```python
from build123d import *

# Parameters (mm, degrees)
SKETCH1_R           = 9
SKETCH1_R_2         = 7
BOSS_EXTRUDE1_DEPTH = 20
BOSS_EXTRUDE2_DEPTH = 9
SKETCH3_R           = 9
SKETCH3_R_2         = 7
BOSS_EXTRUDE4_DEPTH = 20
SKETCH6_R           = 5
BOSS_EXTRUDE7_DEPTH = 10
BOSS_EXTRUDE8_START = 25
SKETCH6_3_R         = 5
BOSS_EXTRUDE8_DEPTH = 10


with BuildPart() as part:
    # Sketch1 → Boss-Extrude1 (new body)
    # profile 1 of 3: a face of its own
    with BuildSketch(Plane(origin=(0, 0, 0), x_dir=(0, 0, -1), z_dir=(1, 0, 0))):
        with BuildLine():
            Line((90, 9), (0, 9))
            ThreePointArc((0, 9), (6.363961031, 6.363961031), (9, 0))
            Line((9, 0), (81, 0))
            ThreePointArc((81, 0), (83.636038969, 6.363961031), (90, 9))
        make_face()
    # profile 2 of 3: a face of its own
    with BuildSketch(Plane(origin=(0, 0, 0), x_dir=(0, 0, -1), z_dir=(1, 0, 0))):
        Circle(SKETCH1_R)
        Circle(SKETCH1_R_2, mode=Mode.SUBTRACT)
    # profile 3 of 3: a face of its own
    with BuildSketch(Plane(origin=(0, 0, 0), x_dir=(0, 0, -1), z_dir=(1, 0, 0))):
        with Locations((90, 0)):
            Circle(SKETCH1_R)
        with Locations((90, 0)):
            Circle(SKETCH1_R_2, mode=Mode.SUBTRACT)
    extrude(amount=-BOSS_EXTRUDE1_DEPTH)

    # Sketch2 → Boss-Extrude2 (add)
    with BuildSketch(Plane(origin=(0, 9, 0), x_dir=(1, 0, 0), z_dir=(0, 1, 0))):
        Polygon((0, 62.5), (50, 62.5), (50, 52.5), (10, 52.5), (10, 37.5), (50, 37.5), (50, 27.5), (0, 27.5), align=None)
    extrude(amount=-BOSS_EXTRUDE2_DEPTH)

    # Sketch3 → Boss-Extrude4 (add)
    # profile 1 of 4: a face of its own
    with BuildSketch(Plane(origin=(50, 0, 0), x_dir=(0, 0, -1), z_dir=(1, 0, 0))):
        Circle(SKETCH3_R)
        Circle(SKETCH3_R_2, mode=Mode.SUBTRACT)
    # profile 2 of 4: a face of its own
    with BuildSketch(Plane(origin=(50, 0, 0), x_dir=(0, 0, -1), z_dir=(1, 0, 0))):
        with BuildLine():
            Line((27.5, 9), (0, 9))
            ThreePointArc((0, 9), (6.363961031, 6.363961031), (9, 0))
            Line((9, 0), (27.5, 0))
            Line((27.5, 0), (27.5, 9))
        make_face()
    # profile 3 of 4: a face of its own
    with BuildSketch(Plane(origin=(50, 0, 0), x_dir=(0, 0, -1), z_dir=(1, 0, 0))):
        with BuildLine():
            Line((90, 9), (52.5, 9))
            Line((52.5, 9), (52.5, 0))
            Line((52.5, 0), (81, 0))
            ThreePointArc((81, 0), (83.636038969, 6.363961031), (90, 9))
        make_face()
    # profile 4 of 4: a face of its own
    with BuildSketch(Plane(origin=(50, 0, 0), x_dir=(0, 0, -1), z_dir=(1, 0, 0))):
        with Locations((90, 0)):
            Circle(SKETCH3_R)
        with Locations((90, 0)):
            Circle(SKETCH3_R_2, mode=Mode.SUBTRACT)
    extrude(amount=-BOSS_EXTRUDE4_DEPTH)

    # Sketch6 → Boss-Extrude7 (add)
    with BuildSketch(Plane.XY.offset(-52.5)):
        with BuildLine():
            Line((10, 0), (24.4, -19.2))
            ThreePointArc((24.4, -19.2), (30, -22), (35.6, -19.2))
            Line((35.6, -19.2), (50, 0))
            Line((50, 0), (10, 0))
        make_face()
        with Locations((30, -15)):
            Circle(SKETCH6_R, mode=Mode.SUBTRACT)
    extrude(amount=-BOSS_EXTRUDE7_DEPTH)

    # Sketch6<3> → Boss-Extrude8 (add)
    with BuildSketch(Plane.XY.offset(-52.5).offset(BOSS_EXTRUDE8_START)):
        with BuildLine():
            Line((10, 0), (24.4, -19.2))
            ThreePointArc((24.4, -19.2), (30, -22), (35.6, -19.2))
            Line((35.6, -19.2), (50, 0))
            Line((50, 0), (10, 0))
        make_face()
        with Locations((30, -15)):
            Circle(SKETCH6_3_R, mode=Mode.SUBTRACT)
    extrude(amount=-BOSS_EXTRUDE8_DEPTH)


solid = part.part
```
Source: CAD feature listing. Evaluate the final solid. Frame: model axes, mm. A direction names the side the tool comes from. Give positions to 0.01 mm unless a question says otherwise; leave off trailing zeros. Loops run counter-clockwise (first coordinate to the right, second up) from the corner with the lowest first, then second, coordinate; pieces in that order, holes last. Notation, with made-up numbers: (-25, 49) -> (34, 49) arc R19 cw to (34, 65) -> close; hole circle Ø11 at (0.5, 36). An arc over 180 degrees is marked (long way). Put each result on its own line as item: value. Start each with the question number.
1) Cut plane B-B (z = -69). Return loops of the section in (x, y), then the cut area to 3 significant figures.
2) Contact query for flat-ended pins moving along their axis: P1, Ø9.5, axis at x = 34.5, y = -11.5, coming from the -Z side; P2, Ø14.5, axis at y = -1.5, z = -3, coming from the +X side; P3, Ø1.5, axis at x = 28, y = -6.5, coming from the +Z side; P4, Ø20.5, axis at x = 37, z = -74, coming from the -Y side. Output: stop coordinate, or through.
3) Reachability of faces 5 (the face through (0, 2, -9)), 6 (the face through (-8, 0, -44)), 7 (the face through (0, 2, -76)) from +Z, -Z, +X, -X, +Y, -Y: full face, straight path, thin tool, end or side. Return the list, or none.
4) Cut plane C-C (x = -2). Return loops of the section in (y, z).
5) Cut plane D-D (x = 23). Return loops of the section in (y, z), then the cut area to 3 significant figures.
6) Material intervals for probe 1 along X at (y, z) = (-7, -3); probe 2 along Y at (x, z) = (-14, -90); probe 3 along Z at (x, y) = (10.5, 4.5), sorted ascending.
7) Draft query along X for faces 1 (the face through (50, 4, -14)), 2 (the face through (25, -3, -62.5)), 3 (the face through (40, 0, -72)), 4 (the face through (17.099, -9.466, -57.43)). Return one class per face: released by +X, released by -X, zero draft, split by the parting line, or undercut.
8) Cut plane A-A (y = -18). Return loops of the section in (x, z), then the cut area to 3 significant figures.
Results are:
1. outline: (-20, 0) -> (0, 0) -> (0, 9) -> (-20, 9) -> close; (30, 0) -> (50, 0) -> (50, 9) -> (30, 9) -> close
1. area: 360 mm2
2. P1: stops at z = -95.95
2. P2: stops at x = 50
2. P3: stops at z = -27.5
2. P4: stops at y = -6.92
3. face 5: +Z, +Y, -Y
3. face 6: -X, -Y
3. face 7: -Z, +Y, -Y
4. outline: (0, -81) arc R9 ccw (long way) to (9, -90) -> (9, 0) arc R9 ccw (long way) to (0, -9) -> close; hole circle Ø14 at (0, -90); hole circle Ø14 at (0, 0)
5. outline: (-17.33, -62.5) -> (9, -62.5) -> (9, -52.5) -> (-17.33, -52.5) -> close; (-17.33, -37.5) -> (9, -37.5) -> (9, -27.5) -> (-17.33, -27.5) -> close
5. area: 527 mm2
6. probe 1: x = -20 to 0, 30 to 50
6. probe 2: y = -9 to -7, 7 to 9
6. probe 3: z = -62.5 to -52.5, -37.5 to -27.5
7. face 1: released by +X
7. face 2: undercut
7. face 3: zero draft
7. face 4: released by -X
8. outline: (23.5, -62.5) -> (26, -62.5) -> (26, -52.5) -> (23.5, -52.5) -> close; (23.5, -37.5) -> (26, -37.5) -> (26, -27.5) -> (23.5, -27.5) -> close; (34, -62.5) -> (36.5, -62.5) -> (36.5, -52.5) -> (34, -52.5) -> close; (34, -37.5) -> (36.5, -37.5) -> (36.5, -27.5) -> (34, -27.5) -> close
8. area: 100 mm2
